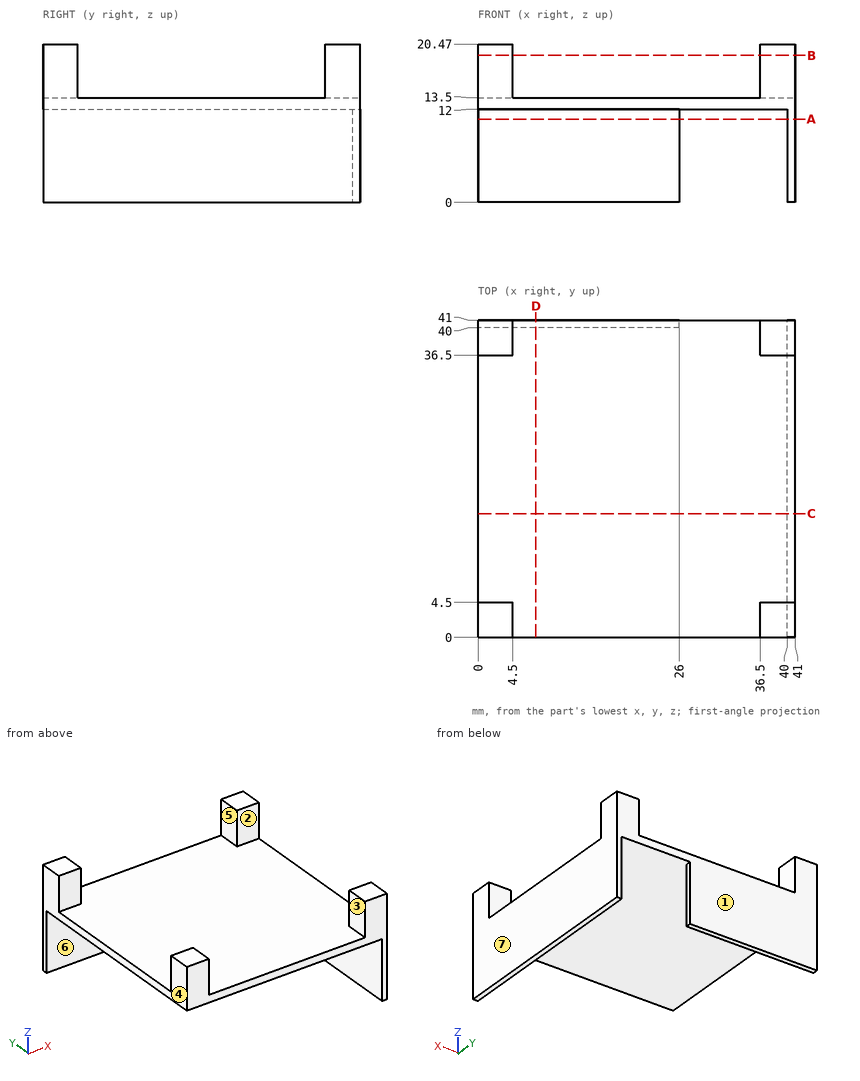
Input: dimensioned drawing with shaded views. Units: mm. Origin: part minimum x, y, z. A direction names the side the tool comes from. Coordinates: 2 decimals unless noted, no trailing zeros. Loops run counter-clockwise (first coordinate to the right, second up) from the corner with the lowest first, then second, coordinate; pieces in that order, holes last. Notation, with made-up numbers: M 16,40.25 L 72,40.25 A25 ccw 72,56.25 Z; hole C 53.25,3 d1. An arc over 180 degrees is marked long. Use a Markdown table: item, result. Add a question column.
1) Section C-C, the plane y = 16. Return the cut outline in (x, z), plus the area to 3 significant figures.
2) Section A-A, the plane z = 10.75. Return the cut outline in (x, y).
3) Draft query along X for the marked faces 4, 5, 6 and 7. Return one class per face: +X half, -X half, draft (parallel to the pull), parting line (faces both ways), or undercut.
4) Set-up query: the marked faces 1, 2 and 3. Return all of +Z, -Z, +X, -X, +Y, -Y with unobstructed straight access to the full face (end or side cutting, diameter ignored); none if empty.
5) Pin query (flat end, axial travel): P1, Ø3.5, axis at x = 38.5, z = 16.5, coming from the -Y side; P2, Ø5, axis at x = 29.5, y = 30.5, coming from the -Z side; P3, Ø1, axis at x = 35, y = 9, coming from the +Z side; P4, Ø5, axis at y = 9, z = 3, coming from the -X side. Return the tip coordinate at first contact, or that it passes through.
6) Line query: L1, parallel to X at y = 39, z = 13.75; L2, parallel to Z at x = 25, y = 34.5; L3, parallel to X at y = 10, z = 3.5. Output: solid intervals per line, ascending. Write a range as from..to.
7) Section B-B, the plane z = 19. Return the cut outline in (x, y).
Answer below:
| question | item | result |
|---|---|---|
| 1 | outline | M 0,12 L 40,12 L 40,0 L 41,0 L 41,13.5 L 0,13.5 Z |
| 1 | area | 73.5 mm2 |
| 2 | outline | M 0,40 L 26,40 L 26,41 L 0,41 Z; M 40,0 L 41,0 L 41,41 L 40,41 Z |
| 3 | face 4 | -X half |
| 3 | face 5 | undercut |
| 3 | face 6 | draft |
| 3 | face 7 | +X half |
| 4 | face 1 | +Z, -Z, +X, -X, +Y |
| 4 | face 2 | +Z, +X, -X |
| 4 | face 3 | +Z, +Y, -Y |
| 5 | P1 | y = 0 |
| 5 | P2 | z = 12 |
| 5 | P3 | z = 13.5 |
| 5 | P4 | x = 40 |
| 6 | L1 | 0..4.5, 36.5..41 |
| 6 | L2 | 12..13.5 |
| 6 | L3 | 40..41 |
| 7 | outline | M 0,0 L 4.5,0 L 4.5,4.5 L 0,4.5 Z; M 0,36.5 L 4.5,36.5 L 4.5,41 L 0,41 Z; M 36.5,0 L 41,0 L 41,4.5 L 36.5,4.5 Z; M 36.5,36.5 L 41,36.5 L 41,41 L 36.5,41 Z |
